Read the model definition and answer for the solid it produces. Units are mm, in the model's axes. A direction names the side the tool comes from. Round coordinates to 2 decimals unless told otherwise and drop trailing zeros. Write each loop counter-clockwise with the first axis right and the second up, starting at its lowest first coordinate (ties: lowest second). Pieces come first, ordered by that corner, then holes. Notation, with made-up numbers: (17.25, 38.25) - (58.25, 38.25) arc R22 ccw to (58.25, 66.25) - close; hole circle Ø2 at (-7.75, -25.75). An arc over 180 degrees is marked (long way). Answer as CSV lines item,"result". Start each with the question number.
1) Find section D-D on x = 15. Determine the outline of the cut face in (y, z).
2) Which of the six approach directions +Z, -Z, +X, -X, +Y, -Y give full straight-line access (tool end or side, diameter ignored) to faces 4 (the flat face through (21, -2, 2)), 5 (the flat face through (2.5, 6, 26)), 6 (the flat face through (21, 0, 0))?
3) Each of these flat-tipped pins is pushed along its axis until it touches: pin 1 (2 mm diameter, centred on y = 6.5, z = 26, fed in from -X); pin 2 (3 mm diameter, centred on x = 21.5, y = 1, fed in from +Z); pin 3 (8 mm diameter, centred on y = 0.5, z = -7.5, fed in from -X). Where does it stop, or does it pass through?
4) Find section C-C on z = 0. Determine the outline of the cut face in (x, y), then the cut area to 3 significant figures.
5) Find section A-A on x = 8. Determine the outline of the cut face in (y, z).
6) For a pull along Z with two mould halves and no side action, classify faces 1 (the cylindrical face through (25.495, 5.916, -0.526)), 2 (the flat face through (2.5, 6, -26)), 3 (the flat face through (30, 8, -2)) as +Z half, -Z half, draft (parallel to the pull), parting line (faces both ways), or undercut.
7) Consider line 1 along Z through (x, y) = (14, 3.25); line 2 along Y through (x, z) = (7, -24); line 3 along Z through (x, y) = (32.5, 14.5). Determine where each line is inside the solid, lowest interval first.
8) Find section B-B on y = 4. Determine the outline of the cut face in (x, z), then the cut area to 3 significant figures.
from build123d import *

# Parameters (mm, degrees)
BOSS_EXTRUDE1_DEPTH = 12
BOSS_EXTRUDE2_START = -2
BOSS_EXTRUDE2_DEPTH = 2
SKETCH4_W           = 6
SKETCH4_H           = 4
BOSS_EXTRUDE3_DEPTH = 20


with BuildPart() as part:
    # Sketch1 → Boss-Extrude1 (new body)
    with BuildSketch(Plane(origin=(0, 0, 0), x_dir=(1, 0, 0), z_dir=(0, 1, 0))):
        with BuildLine():
            Line((2.5, 27.386127875), (2.5, 25.377155081))
            ThreePointArc((2.5, 25.377155081), (25.5, 0), (2.5, -25.377155081))
            Line((2.5, -25.377155081), (2.5, -27.386127875))
            ThreePointArc((2.5, -27.386127875), (27.5, 0), (2.5, 27.386127875))
        make_face()
    extrude(amount=BOSS_EXTRUDE1_DEPTH)

    # Sketch2 → Boss-Extrude2 (add)
    with BuildSketch(Plane(origin=(0, 0, 0), x_dir=(1, 0, 0), z_dir=(0, 1, 0)).offset(BOSS_EXTRUDE2_START)):
        with BuildLine():
            Line((2.5, 27.386127875), (1.863636364, 20.415113507))
            ThreePointArc((1.863636364, 20.415113507), (20.5, 0), (1.863636364, -20.415113507))
            Line((1.863636364, -20.415113507), (2.5, -27.386127875))
            ThreePointArc((2.5, -27.386127875), (27.5, 0), (2.5, 27.386127875))
        make_face()
    extrude(amount=BOSS_EXTRUDE2_DEPTH)

    # Sketch4 → Boss-Extrude3 (add)
    with BuildSketch(Plane(origin=(0, -2, 0), x_dir=(1, 0, 0), z_dir=(0, 1, 0))):
        with Locations((30, 0)):
            Rectangle(SKETCH4_W, SKETCH4_H)
    extrude(amount=BOSS_EXTRUDE3_DEPTH)


solid = part.part
Check values:
1,outline,"(-2, -23.05) - (12, -23.05) - (12, -20.62) - (0, -20.62) - (0, -13.97) - (-2, -13.97) - close; (-2, 13.97) - (0, 13.97) - (0, 20.62) - (12, 20.62) - (12, 23.05) - (-2, 23.05) - close"
2,face 4,"+Z, -Z, +X, -X, -Y"
2,face 5,"+Z, -Z, -X, +Y"
2,face 6,"-X, +Y"
3,pin 1,"stops at x = 2.5"
3,pin 2,"stops at z = 18.87"
3,pin 3,"stops at x = 16.99"
4,outline,"(20.5, -2) - (33, -2) - (33, 18) - (27, 18) - (27, 12) - (25.5, 12) - (25.5, 0) - (20.5, 0) - close"
4,area,"151 mm^2"
5,outline,"(-2, -26.31) - (12, -26.31) - (12, -24.21) - (0, -24.21) - (0, -18.87) - (-2, -18.87) - close; (-2, 18.87) - (0, 18.87) - (0, 24.21) - (12, 24.21) - (12, 26.31) - (-2, 26.31) - close"
6,face 1,"undercut"
6,face 2,"draft"
6,face 3,"-Z half"
7,line 1,"z = -23.67 to -21.31, 21.31 to 23.67"
7,line 2,"y = -2 to 0"
7,line 3,"z = -2 to 2"
8,outline,"(2.5, -27.39) arc R27.5 ccw to (27.43, -2) - (33, -2) - (33, 2) - (27.43, 2) arc R27.5 ccw to (2.5, 27.39) - (2.5, 25.38) arc R25.5 cw to (2.5, -25.38) - close"
8,area,"179 mm^2"
